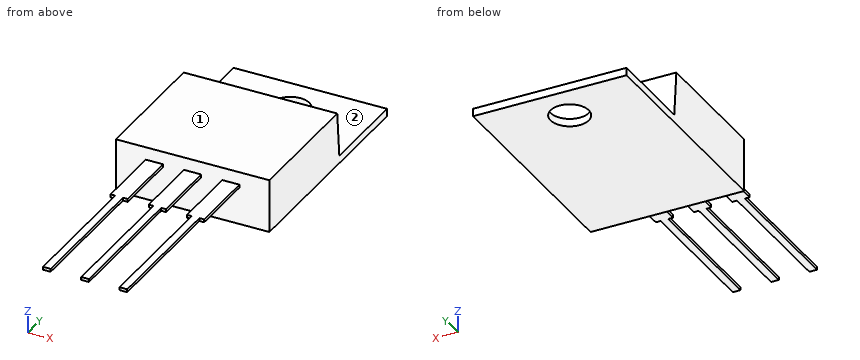
from build123d import *

# Parameters (mm, degrees)
SKETCH1_W           = 10.2
SKETCH1_H           = 15
BOSS_EXTRUDE1_DEPTH = 0.51
SKETCH2_W           = 10.2
SKETCH2_H           = 8.65
BOSS_EXTRUDE2_DEPTH = 3.04
DRAFT1_ANGLE        = 5
SKETCH3_W           = 0.2
SKETCH3_H           = 4.5
EXTRUDE_THIN1_DEPTH = 0.57
SKETCH4_W           = 0.2
SKETCH4_H           = 9.22
EXTRUDE_THIN2_DEPTH = 0.255
LPATTERN1_COUNT     = 3
LPATTERN1_PITCH     = 2.54
CUT_EXTRUDE1_REACH  = 2.51
SKETCH5_R           = 1.27


with BuildPart() as part:
    # Sketch1 → Boss-Extrude1 (new body)
    with BuildSketch(Plane.XY):
        with Locations((5.1, 7.5)):
            Rectangle(SKETCH1_W, SKETCH1_H)
    extrude(amount=BOSS_EXTRUDE1_DEPTH)

    # Sketch2 → Boss-Extrude2 (add)
    with BuildSketch(Plane.XY.offset(0.51)):
        with Locations((5.1, 4.325)):
            Rectangle(SKETCH2_W, SKETCH2_H)
    extrude(amount=BOSS_EXTRUDE2_DEPTH)

    # Draft1
    draft1_faces = [part.faces().sort_by_distance(p)[0] for p in [
        (5.1, 8.65, 2.03),
    ]]
    draft(draft1_faces, Plane.XY.offset(3.55), DRAFT1_ANGLE)

    # Sketch3 → Extrude-Thin1 (add, symmetric)
    with BuildSketch(Plane.ZY.offset(-2.56)):
        with Locations((2.6, -2.25)):
            Rectangle(SKETCH3_W, SKETCH3_H)
    extrude_thin1 = extrude(amount=EXTRUDE_THIN1_DEPTH, both=True)

    # Sketch4 → Extrude-Thin2 (add, symmetric)
    with BuildSketch(Plane.ZY.offset(-2.56)):
        with Locations((2.6, -9.11)):
            Rectangle(SKETCH4_W, SKETCH4_H)
    extrude_thin2 = extrude(amount=EXTRUDE_THIN2_DEPTH, both=True)

    # LPattern1: Extrude-Thin1, Extrude-Thin2 ×3
    with Locations(*[(i * LPATTERN1_PITCH, 0, 0) for i in range(1, LPATTERN1_COUNT)]):
        add(extrude_thin1)
        add(extrude_thin2)

    # Sketch5 → Cut-Extrude1 (cut, up to next)
    with BuildSketch(Plane.XY.offset(0.51), mode=Mode.PRIVATE) as cut_extrude1_sk1:
        with Locations((5.1, 12.46)):
            Circle(SKETCH5_R)
    cut_extrude1_tool1 = extrude(cut_extrude1_sk1.sketch, amount=-CUT_EXTRUDE1_REACH, mode=Mode.PRIVATE) & part.part
    add(cut_extrude1_tool1.solids().sort_by_distance((5.1, 12.46, 0.51))[0], mode=Mode.SUBTRACT)


solid = part.part
Could you check a few things on this model? Use its own coordinates, in mm. Face numbers are marked on the shaded views. A direction names the side the tool comes from. Give positions to 0.01 mm unless a question says otherwise; leave off trailing zeros. Order: outer loops, then holes, each group sorted by start corner. A loop starts at its lowest first (then second) coordinate and runs counter-clockwise, first axis right, second up.
Item 1: If we section it at D-D, the plane x = 1: Write out the boundary of the cut face in (y, z), plus the area to 3 significant figures.
Item 2: If we section it at A-A, the plane x = 5.1: Write out the boundary of the cut face in (y, z).
Item 3: If we section it at B-B, the plane y = -10.25: Write out the boundary of the cut face in (x, z) (3 decimals), plus the area to 3 significant figures.
Item 4: If we section it at C-C, the plane y = 12.46: Write out the boundary of the cut face in (x, z).
Item 5: For the marked faces 1 and 2, which set-ups out of +Z, -Z, +X, -X, +Y, -Y let a thin tool reach every point of the face, with its end or its side?
Item 6: I need wall thicknesses on line 1 (Y direction, x = 5.1, z = 0.1); line 2 (Z direction, x = 6.75, y = 9.75); line 3 (Y direction, x = 6, z = 2.85). Which ranges of each line are inside material? Lowest first, please.
Item 7: I'm going to push flat-ended pins straight in: pin 1 (0.9 mm diameter, centred on x = 5, y = -9, fed in from +Z); pin 2 (1.8 mm diameter, centred on x = 6, y = 12, fed in from +Z); pin 3 (1.5 mm diameter, centred on y = -7, z = 3, fed in from -X) (3 decimals). Where does each tip first touch, or does it pass through?
Values:
1. outline: (0, 0) - (15, 0) - (15, 0.51) - (8.92, 0.51) - (8.65, 3.55) - (0, 3.55) - close
1. area: 34.4 mm2
2. outline: (-13.72, 2.5) - (0, 2.5) - (0, 0) - (11.19, 0) - (11.19, 0.51) - (8.92, 0.51) - (8.65, 3.55) - (0, 3.55) - (0, 2.7) - (-13.72, 2.7) - close; (13.73, 0) - (15, 0) - (15, 0.51) - (13.73, 0.51) - close
3. outline: (2.305, 2.5) - (2.815, 2.5) - (2.815, 2.7) - (2.305, 2.7) - close; (4.845, 2.5) - (5.355, 2.5) - (5.355, 2.7) - (4.845, 2.7) - close; (7.385, 2.5) - (7.895, 2.5) - (7.895, 2.7) - (7.385, 2.7) - close
3. area: 0.306 mm2
4. outline: (0, 0) - (3.83, 0) - (3.83, 0.51) - (0, 0.51) - close; (6.37, 0) - (10.2, 0) - (10.2, 0.51) - (6.37, 0.51) - close
5. face 1: +Z, +X, -X, +Y, -Y
5. face 2: +Z, +X, -X, +Y
6. line 1: y = 0 to 11.19, 13.73 to 15
6. line 2: z = 0 to 0.51
6. line 3: y = 0 to 8.71
7. pin 1: stops at z = 2.7
7. pin 2: stops at z = 0.51
7. pin 3: stops at x = 2.305
